```python
from build123d import *

# Parameters (mm, degrees)
SKETCH_R     = 2
PAD_DEPTH    = 3
SKETCH001_W  = 4.15
SKETCH001_H  = 115
PAD001_DEPTH = 11.7
SKETCH002_R  = 2
SKETCH002_W  = 80
SKETCH002_H  = 6
POCKET_DEPTH = 15
SKETCH003_W  = 4.09
SKETCH003_H  = 115
PAD002_DEPTH = 3.5
FILLET_R     = 2
FILLET001_R  = 2
FILLET002_R  = 2
FILLET003_R  = 2


with BuildPart() as part:
    # Sketch → Pad (new body)
    with BuildSketch(Plane.XY):
        with BuildLine():
            Line((-14.5, 57.5), (14.5, 57.5))
            ThreePointArc((17.5, 54.5), (16.62132, 56.62132), (14.5, 57.5))
            Line((17.5, 54.5), (17.5, 45.5))
            ThreePointArc((14.5, 42.5), (16.62132, 43.37868), (17.5, 45.5))
            Line((14.5, 42.5), (5, 42.5))
            Line((5, 42.5), (5, -42.5))
            Line((5, -42.5), (14.5, -42.5))
            ThreePointArc((17.5, -45.5), (16.62132, -43.37868), (14.5, -42.5))
            Line((17.5, -45.5), (17.5, -54.5))
            ThreePointArc((14.5, -57.5), (16.62132, -56.62132), (17.5, -54.5))
            Line((14.5, -57.5), (-14.5, -57.5))
            ThreePointArc((-17.5, -54.5), (-16.62132, -56.62132), (-14.5, -57.5))
            Line((-17.5, -54.5), (-17.5, -45.5))
            ThreePointArc((-14.5, -42.5), (-16.62132, -43.37868), (-17.5, -45.5))
            Line((-5, -42.5), (-14.5, -42.5))
            Line((-5, 42.5), (-5, -42.5))
            Line((-14.5, 42.5), (-5, 42.5))
            ThreePointArc((-17.5, 45.5), (-16.62132, 43.37868), (-14.5, 42.5))
            Line((-17.5, 45.5), (-17.5, 54.5))
            ThreePointArc((-14.5, 57.5), (-16.62132, 56.62132), (-17.5, 54.5))
        make_face()
        with Locations((-10, 50)):
            Circle(SKETCH_R, mode=Mode.SUBTRACT)
        with Locations((10, 50)):
            Circle(SKETCH_R, mode=Mode.SUBTRACT)
        with Locations((-10, -50)):
            Circle(SKETCH_R, mode=Mode.SUBTRACT)
        with Locations((10, -50)):
            Circle(SKETCH_R, mode=Mode.SUBTRACT)
    extrude(amount=PAD_DEPTH)

    # Sketch001 → Pad001 (join)
    with BuildSketch(Plane.XY.offset(3)):
        with Locations((-2.925, 0)):
            Rectangle(SKETCH001_W, SKETCH001_H)
        with Locations((2.925, 0)):
            Rectangle(SKETCH001_W, SKETCH001_H)
    extrude(amount=PAD001_DEPTH)

    # Sketch002 → Pocket (cut)
    with BuildSketch(Plane.YZ.offset(5)):
        with Locations((-46.5, 11.5)):
            Circle(SKETCH002_R)
        with Locations((46.5, 11.5)):
            Circle(SKETCH002_R)
        with Locations((0, 12)):
            Rectangle(SKETCH002_W, SKETCH002_H)
    extrude(amount=-POCKET_DEPTH, mode=Mode.SUBTRACT)

    # Sketch003 → Pad002 (join)
    with BuildSketch(Plane.XY.offset(3)):
        with Locations((0.341939, 0)):
            Rectangle(SKETCH003_W, SKETCH003_H)
    extrude(amount=PAD002_DEPTH)

    # Fillet
    fillet_edges = [part.edges().sort_by_distance(p)[0] for p in [
        (2.925, -57.5, 14.7),
    ]]
    fillet(fillet_edges, radius=FILLET_R)

    # Fillet001
    fillet001_edges = [part.edges().sort_by_distance(p)[0] for p in [
        (-2.925, -57.5, 14.7),
    ]]
    fillet(fillet001_edges, radius=FILLET001_R)

    # Fillet002
    fillet002_edges = [part.edges().sort_by_distance(p)[0] for p in [
        (-2.925, 57.5, 14.7),
        (2.925, 57.5, 14.7),
    ]]
    fillet(fillet002_edges, radius=FILLET002_R)

    # Fillet003
    fillet003_edges = [part.edges().sort_by_distance(p)[0] for p in [
        (-2.925, -40, 14.7),
        (2.925, -40, 14.7),
        (-2.925, 40, 14.7),
        (2.925, 40, 14.7),
    ]]
    fillet(fillet003_edges, radius=FILLET003_R)


solid = part.part
```
Could you check a few things on this model? Use its own coordinates, in mm. A direction names the side the tool comes from. Coordinates: 2 decimals unless noted, no trailing zeros. Order: outer loops, then holes, each group sorted by start corner. A loop starts at its lowest first (then second) coordinate and runs counter-clockwise, first axis right, second up. Notation, with made-up numbers: M -31,21.5 L -1,21.5 A28 cw -1,40.5 Z; hole C 38.25,6 d8. An arc over 180 degrees is marked long. Use one line per item in the form item = value. Start each with the question number.
1. Please list where these lines run through material, in increasing order: line 1 (Y direction, x = -10, z = 1.1); line 2 (X direction, y = -39.5, z = 8.5); line 3 (Z direction, x = 3.35, y = 46.5).
2. For pin 1 (4 mm diameter, centred on x = 11, y = -53.5, fed in from +Z); pin 2 (1.5 mm diameter, centred on y = -1.5, z = 3, fed in from +X); pin 3 (0.5 mm diameter, centred on x = 0.5, y = -0.5, fed in from +Z), each with a flat end and sliding along its axis, tell me the tip position at first contact or that it passes through.
3. Suppose I cut it at B-B on y = -50. Write out the boundary of the cut face in (x, z).
4. Suppose I cut it at A-A on x = 10. Write out the boundary of the cut face in (y, z), then the cut area to 3 significant figures.
5. Suppose I cut it at D-D on x = 3. Write out the boundary of the cut face in (y, z).
6. We'd pull the mould along X, two halves only. Please class faces 6 (the cylindrical face through (-2.9, -56.93, 14.1)), 7 (the cylindrical face through (10.923, 48.226, 1.479)), 8 (the cylindrical face through (-16.6, 56.64, 1.48)): +X half, -X half, draft (parallel to the pull), parting line (faces both ways), or undercut.
7. Suppose I cut it at C-C on z = 11.5. Count the separate pieces of the cut face and the enclosed holes in it, then the cut area to 3 significant figures.
8. On a 3-axis mill with a long thin cutter (end or side, diameter ignored), from which of +Z, -Z, +X, -X, +Y, -Y can I reach the whole of each face in a straight line? I mean faces 1 (the cylindrical face through (-2.896, -46.76, 13.483)), 2 (the cylindrical face through (-16.6, -43.36, 1.48)), 3 (the flat face through (13, -50, 3)), 4 (the cylindrical face through (2.9, -40.6, 14.13)), 5 (the cylindrical face through (16.64, -43.4, 1.48)). Say none if no direction works.
Geometry says:
q1.line_1 = -57.5 to -52, -48 to -42.5, 42.5 to 48, 52 to 57.5
q1.line_2 = -5 to -0.85, 0.85 to 5
q1.line_3 = 0 to 9.5, 13.5 to 14.7
q2.pin_1 = 3
q2.pin_2 = 5
q2.pin_3 = 6.5
q3.outline = M -17.5,0 L -12,0 L -12,3 L -17.5,3 Z; M -8,0 L 8,0 L 8,3 L 5,3 L 5,14.7 L 0.85,14.7 L 0.85,6.5 L -0.85,6.5 L -0.85,14.7 L -5,14.7 L -5,3 L -8,3 Z; M 12,0 L 17.5,0 L 17.5,3 L 12,3 Z
q4.outline = M -57.5,0 L -52,0 L -52,3 L -57.5,3 Z; M -48,0 L -42.5,0 L -42.5,3 L -48,3 Z; M 42.5,0 L 48,0 L 48,3 L 42.5,3 Z; M 52,0 L 57.5,0 L 57.5,3 L 52,3 Z
q4.area = 66.0 mm^2
q5.outline = M -57.5,0 L 57.5,0 L 57.5,12.7 A2 ccw 55.5,14.7 L 42,14.7 A2 ccw 40,12.7 L 40,9 L -40,9 L -40,12.7 A2 ccw -42,14.7 L -55.5,14.7 A2 ccw -57.5,12.7 Z; hole C -46.5,11.5 d4; hole C 46.5,11.5 d4
q6.face_6 = draft
q6.face_7 = undercut
q6.face_8 = -X half
q7.separate_pieces = 8
q7.enclosed_holes = 0
q7.area = 224 mm^2
q8.face_1 = +X, -X
q8.face_2 = +Z, -Z, -X
q8.face_3 = +Z, +X, +Y, -Y
q8.face_4 = +Z, +X, -X
q8.face_5 = +Z, -Z, +X
